```python
from build123d import *

# Parameters (mm, degrees)
FLANGE_HOLES_D    = 2.8702
DOWEL_HOLES_D     = 4.7625
DOWEL_HOLES_DEPTH = 6.35
DOWEL_HOLES_TIP   = 1.430799349
FILLET1_R         = 8.89
CHAMFER1_SIZE     = 2.141545552
CHAMFER1_SIZE_2   = 2.54


with BuildPart() as part:
    # Sketch2 → Main Structure (revolve)
    with BuildSketch(Plane.XY, mode=Mode.PRIVATE) as main_structure_sk:
        Polygon((0, 20.583496156), (0, 56.388), (9.525, 56.388), (9.525, 16.256), (66.806461084, 16.256), (139.7, 31.75), (139.7, 29.592458901), (60.325, 12.720781818), (60.325, 14.351), (10.795, 14.351), align=None)
    revolve(main_structure_sk.sketch.rotate(Axis((0, 0, 0), (1, 0, 0)), 90), axis=Axis((0, 0, 0), (1, 0, 0)))

    # Flange Holes (through all)
    with Locations(Plane.ZY):
        with Locations((0, -51.6255), (-25.81275, -44.708994483), (-44.708994483, -25.81275), (-51.6255, 0), (-44.708994483, 25.81275), (-25.81275, 44.708994483), (0, 51.6255), (25.81275, 44.708994483), (44.708994483, 25.81275), (51.6255, 0), (44.708994483, -25.81275), (25.81275, -44.708994483)):
            Hole(FLANGE_HOLES_D / 2)

    # Dowel Holes
    with Locations(Plane.ZY):
        with Locations((49.866403745, -13.361662613), (-49.866403745, 13.361662613)):
            Hole(DOWEL_HOLES_D / 2, depth=DOWEL_HOLES_DEPTH)
            with Locations((0, 0, -(DOWEL_HOLES_DEPTH + DOWEL_HOLES_TIP / 2))):  # 118° drill point
                Cone(0, DOWEL_HOLES_D / 2, DOWEL_HOLES_TIP, mode=Mode.SUBTRACT)

    # Fillet1
    fillet1_edges = [part.edges().sort_by_distance(p)[0] for p in [
        (66.806461084, 0, -16.256),
        (9.525, 0, -16.256),
    ]]
    fillet(fillet1_edges, radius=FILLET1_R)

    # Sketch13 → Cut-Revolve1 (revolve, cut)
    with BuildSketch(Plane(origin=(0, 0, 0), x_dir=(1, 0, 0), z_dir=(0, 1, 0)), mode=Mode.PRIVATE) as cut_revolve1_sk:
        Polygon((0, 38.1), (3.33331808, 0), (0, 0), align=None)
    revolve(cut_revolve1_sk.sketch.rotate(Axis((3.33331808, 0, 0), (-1, 0, 0)), 180), axis=Axis((3.33331808, 0, 0), (-1, 0, 0)), mode=Mode.SUBTRACT)

    # Chamfer1
    # the kernel refuses this chamfer: 3.297690964, 2.54, 2.141545552 mm, written as the material it takes off along each edge
    with BuildSketch(Plane(origin=(139.7, 0, 0), x_dir=(0, 0, 1), z_dir=(0, 1, 0))) as chamfer1_piece_1:
        Polygon((31.75 - CHAMFER1_SIZE * 0.207911690799, -CHAMFER1_SIZE * 0.978147600645), (31.75 - CHAMFER1_SIZE_2, 0), (31.75, 0), align=None)
    revolve(axis=Axis((139.7, 0, 0), (1, 0, 0)), mode=Mode.SUBTRACT)


solid = part.part
```
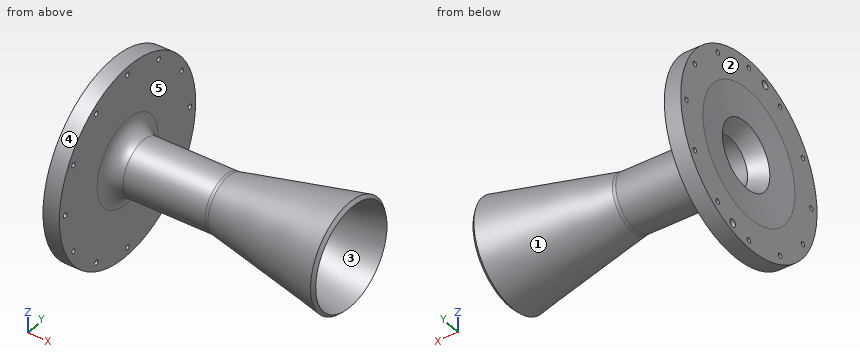
Part model, mm, in its own coordinate system. Face numbers are marked on the shaded views. A direction names the side the tool comes from. Round coordinates to 2 decimals unless told otherwise and drop trailing zeros. Order: outer loops, then holes, each group sorted by start corner. A loop starts at its lowest first (then second) coordinate and runs counter-clockwise, first axis right, second up. Notation, with made-up numbers: M 40,66.25 L 45,66.25 A17 cw 45,74.25 Z; hole C 35,52 d9. An arc over 180 degrees is marked long. Put each result on its own line as item: value. Start each with the question number.
1. Drop flat-ended pins along their axis: pin 1 (2.5 mm diameter, centred on y = -44.71, z = -25.81, fed in from +X); pin 2 (4.5 mm diameter, centred on y = -44.71, z = 25.81, fed in from +X) (3 decimals); pin 3 (4 mm diameter, centred on y = 4, z = -25, fed in from -X); pin 4 (10 mm diameter, centred on x = 27, z = 3.5, fed in from +Y). Give the stop position or say it passes through.
2. Tool access for the marked faces 4 and 5: list every direction of +Z, -Z, +X, -X, +Y, -Y with a clear straight run to the whole face (end or side of a thin tool).
3. Slice it at B-B on x = 92. List the corners of the cut face in (y, z), then the cut area to 3 significant figures.
4. Drill centre lines: probe 1 along Y at (x, z) = (50.5, 0); probe 2 along Y at (x, z) = (3.75, 0); probe 3 along Y at (x, z) = (105.5, 19.5). Where is each one in solid material? Low to high. Write a range as [from, to].
5. Two-plate mould, pull along Z, no slides. Class the marked faces 1, 2 and 3: +Z half, -Z half, draft (parallel to the pull), parting line (faces both ways), or undercut.
6. Slice it at A-A on x = 40.5. List the corners of the cut face in (y, z).
Findings:
1. pin 1: through
1. pin 2: x = 9.525
1. pin 3: x = 0.94
1. pin 4: y = 16.26
2. face 4: +X, -X
2. face 5: none
3. outline: C 0,0 d43.22; hole C 0,0 d38.91
3. area: 278 mm2
4. probe 1: [-16.26, -14.35], [14.35, 16.26]
4. probe 2: [-56.39, -53.06], [-50.19, -18.42], [18.42, 50.19], [53.06, 56.39]
4. probe 3: [-14.8, -10.87], [10.87, 14.8]
5. face 1: parting line
5. face 2: draft
5. face 3: undercut
6. outline: C 0,0 d32.51; hole C 0,0 d28.7
